Read the model definition and answer for the solid it produces. Units are mm, in the model's axes. Coordinates: 2 decimals unless noted, no trailing zeros. Order: outer loops, then holes, each group sorted by start corner. A loop starts at its lowest first (then second) coordinate and runs counter-clockwise, first axis right, second up. Notation, with made-up numbers: M -3,61.25 L 53,61.25 A22 cw 53,74.25 Z; hole C 7,64 d8. An arc over 180 degrees is marked long. Use a Markdown table: item, result. Add a question column.
1) Find section C-C on x = -18.5. Count the separate pieces of the cut face and the enclosed holes in it, plus the area to 3 significant figures.
2) Find the intervals of material crossed by probe 1 along X at (y, z) = (1.85, -2); probe 2 along X at (y, z) = (0.75, -46.5); probe 3 along Z at (x, y) = (48, 1.7), in increasing order. Write a range as [from, to].
3) Find section A-A on z = 0. Write down the section's boundary in (x, y).
4) Find section B-B on x = -57.5. Write down the section's boundary in (y, z).
5) Each of these flat-tipped pins is pushed along its axis until it touches: pin 1 Ø1 at (x, y) = (22, 1) entering from -Z; pin 2 Ø8 at (x, z) = (-49, 46.5) entering from -Y; pin 3 Ø1 at (y, z) = (1, -41.5) entering from -X; pin 4 Ø1 at (y, z) = (1, 49) entering from -X. Where does it stop, or does it pass through?
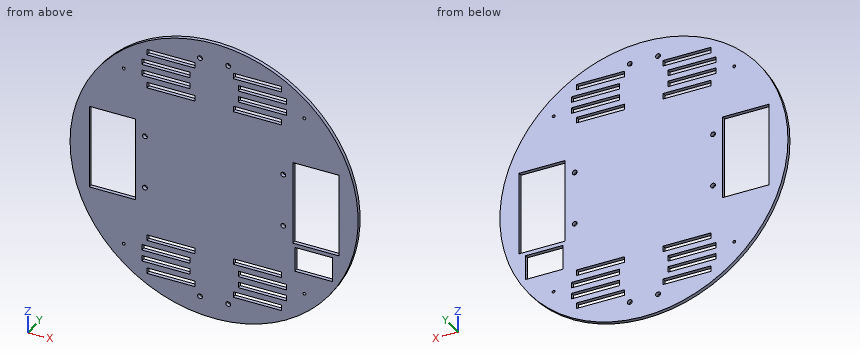
Autodesk Inventor part; units mm, degrees
ref_plane "YZ Plane" through (0, 0, 0) normal (1, 0, 0) x (0, 1, 0)
ref_plane "XZ Plane" through (0, 0, 0) normal (0, 1, 0) x (-1, 0, 0)
ref_plane "XY Plane" through (0, 0, 0) normal (0, 0, 1) x (1, 0, 0)
sketch "Boceto1" plane through (0, 0, 0) normal (0, 1, 0) x (-1, 0, 0)
  circle A0 centre (0, 0) radius 75
  line L0 (65, -22) -> (41, -22)
  line L1 (41, -22) -> (41, 22)
  line L2 (41, 22) -> (65, 22)
  line L3 (65, 22) -> (65, -22)
  line L4 (37.6072, -48.4982) -> (12.6072, -48.4982)
  line L5 (12.6072, -48.4982) -> (12.6072, -45.4982)
  line L6 (12.6072, -45.4982) -> (37.6072, -45.4982)
  line L7 (37.6072, -45.4982) -> (37.6072, -48.4982)
  line L8 (37.6072, -54.4982) -> (12.6072, -54.4982)
  line L9 (12.6072, -54.4982) -> (12.6072, -51.4982)
  line L10 (12.6072, -51.4982) -> (37.6072, -51.4982)
  line L11 (37.6072, -51.4982) -> (37.6072, -54.4982)
  line L12 (35, -60.4982) -> (10, -60.4982)
  line L13 (10, -60.4982) -> (10, -57.4982)
  line L14 (10, -57.4982) -> (35, -57.4982)
  line L15 (35, -57.4982) -> (35, -60.4982)
  line L16 (35, -42.4982) -> (10, -42.4982)
  line L17 (10, -42.4982) -> (10, -39.4982)
  line L18 (10, -39.4982) -> (35, -39.4982)
  line L19 (35, -39.4982) -> (35, -42.4982)
  line L20 (-37.6072, -48.4982) -> (-12.6072, -48.4982)
  line L21 (-12.6072, -48.4982) -> (-12.6072, -45.4982)
  line L22 (-12.6072, -45.4982) -> (-37.6072, -45.4982)
  line L23 (-37.6072, -45.4982) -> (-37.6072, -48.4982)
  line L24 (-37.6072, -54.4982) -> (-12.6072, -54.4982)
  line L25 (-37.6072, -51.4982) -> (-37.6072, -54.4982)
  line L26 (-12.6072, -51.4982) -> (-37.6072, -51.4982)
  line L27 (-12.6072, -54.4982) -> (-12.6072, -51.4982)
  line L28 (-35, -60.4982) -> (-10, -60.4982)
  line L29 (-35, -57.4982) -> (-35, -60.4982)
  line L30 (-10, -57.4982) -> (-35, -57.4982)
  line L31 (-10, -60.4982) -> (-10, -57.4982)
  line L32 (-35, -42.4982) -> (-10, -42.4982)
  line L33 (-35, -39.4982) -> (-35, -42.4982)
  line L34 (-10, -39.4982) -> (-35, -39.4982)
  line L35 (-10, -42.4982) -> (-10, -39.4982)
  line L36 (-65, -22) -> (-41, -22)
  line L37 (-41, -22) -> (-41, 22)
  line L38 (-41, 22) -> (-65, 22)
  line L39 (-65, 22) -> (-65, -22)
  line L40 (37.6072, 49.7986) -> (12.6072, 49.7986)
  line L41 (12.6072, 49.7986) -> (12.6072, 46.7986)
  line L42 (12.6072, 46.7986) -> (37.6072, 46.7986)
  line L43 (37.6072, 46.7986) -> (37.6072, 49.7986)
  line L44 (37.6072, 55.7986) -> (12.6072, 55.7986)
  line L45 (37.6072, 52.7986) -> (37.6072, 55.7986)
  line L46 (12.6072, 52.7986) -> (37.6072, 52.7986)
  line L47 (12.6072, 55.7986) -> (12.6072, 52.7986)
  line L48 (35, 61.7986) -> (10, 61.7986)
  line L49 (35, 58.7986) -> (35, 61.7986)
  line L50 (10, 58.7986) -> (35, 58.7986)
  line L51 (10, 61.7986) -> (10, 58.7986)
  line L52 (35, 43.7986) -> (10, 43.7986)
  line L53 (35, 40.7986) -> (35, 43.7986)
  line L54 (10, 40.7986) -> (35, 40.7986)
  line L55 (10, 43.7986) -> (10, 40.7986)
  line L56 (-35, 40.7986) -> (-35, 43.7986)
  line L57 (-10, 43.7986) -> (-10, 40.7986)
  line L58 (-10, 40.7986) -> (-35, 40.7986)
  line L59 (-35, 43.7986) -> (-10, 43.7986)
  line L60 (-12.6072, 49.7986) -> (-12.6072, 46.7986)
  line L61 (-12.6072, 46.7986) -> (-37.6072, 46.7986)
  line L62 (-37.6072, 46.7986) -> (-37.6072, 49.7986)
  line L63 (-37.6072, 49.7986) -> (-12.6072, 49.7986)
  line L64 (-12.6072, 55.7986) -> (-12.6072, 52.7986)
  line L65 (-12.6072, 52.7986) -> (-37.6072, 52.7986)
  line L66 (-37.6072, 55.7986) -> (-12.6072, 55.7986)
  line L67 (-10, 58.7986) -> (-35, 58.7986)
  line L68 (-35, 61.7986) -> (-10, 61.7986)
  line L69 (-10, 61.7986) -> (-10, 58.7986)
  line L70 (-37.6072, 52.7986) -> (-37.6072, 55.7986)
  line L71 (-35, 58.7986) -> (-35, 61.7986)
  point P0 (0, 25.3749)
  dimension "d0" = 150
  dimension "d1" = 24
  dimension "d2" = 44
  dimension "d3" = 10
  dimension "d4" = 25
  dimension "d5" = 3
  dimension "d6" = 25
  dimension "d7" = 3
  dimension "d8" = 25
  dimension "d9" = 3
  dimension "d10" = 25
  dimension "d11" = 3
  dimension "d12" = 3
  dimension "d13" = 3
  dimension "d14" = 3
  dimension "d15" = 0
extrude "Extrusión1" add sketch "Boceto1" along normal blind 2
sketch "Boceto2" plane through (0, 2, 0) normal (0, 1, 0) x (1, 0, 0)
  line L0 (0, 0) -> (0, -9.9603)
  line L1 (0, 0) -> (61.7788, -62.8893)
  circle A0 centre (47.0174, -47.8626) radius 0.75
  arc A1 (50.5529, -44.327) -> (43.5135, -51.4295) centre (47.0174, -47.8626) ccw
  line L2 (-72.438, 0) -> (-75, 0)
  circle A2 centre (0, 0) radius 72.438
  line L3 (44.0781, -44.8705) -> (47.0174, -47.8626)
  line L4 (43.4505, -51.3665) -> (48.0344, -55.9504)
  line L5 (43.4505, -51.3665) -> (49.9332, -51.3665) construction
  line L6 (47.0174, -47.8626) -> (52.0174, -47.8626) construction
  line L7 (50.5529, -44.327) -> (55.1054, -48.8795)
  line L8 (55.1054, -48.8795) -> (48.0344, -55.9504)
  circle A3 centre (-47.0174, -47.8626) radius 0.75
  arc A4 (-43.5135, -51.4295) -> (-50.5529, -44.327) centre (-47.0174, -47.8626) ccw
  line L9 (-44.0781, -44.8705) -> (-47.0174, -47.8626)
  line L10 (-43.4505, -51.3665) -> (-48.0344, -55.9504)
  line L11 (-43.4505, -51.3665) -> (-49.9332, -51.3665) construction
  line L12 (-47.0174, -47.8626) -> (-52.0174, -47.8626) construction
  line L13 (-50.5529, -44.327) -> (-55.1054, -48.8795)
  line L14 (-55.1054, -48.8795) -> (-48.0344, -55.9504)
  line L15 (0, 0) -> (7.916, 0)
  line L16 (-44.0781, 44.8705) -> (-47.0174, 47.8626)
  circle A5 centre (-47.0174, 47.8626) radius 0.75
  line L17 (-43.4505, 51.3665) -> (-49.9332, 51.3665) construction
  arc A6 (-50.5529, 44.327) -> (-43.5135, 51.4295) centre (-47.0174, 47.8626) ccw
  line L18 (-43.4505, 51.3665) -> (-48.0344, 55.9504)
  line L19 (-47.0174, 47.8626) -> (-52.0174, 47.8626) construction
  line L20 (-50.5529, 44.327) -> (-55.1054, 48.8795)
  line L21 (-55.1054, 48.8795) -> (-48.0344, 55.9504)
  line L22 (0, 0) -> (61.7788, 62.8893)
  circle A7 centre (0, 0) radius 72.438
  circle A8 centre (47.0174, 47.8626) radius 0.75
  arc A9 (43.5135, 51.4295) -> (50.5529, 44.327) centre (47.0174, 47.8626) ccw
  line L23 (44.0781, 44.8705) -> (47.0174, 47.8626)
  line L24 (43.4505, 51.3665) -> (48.0344, 55.9504)
  line L25 (47.0174, 47.8626) -> (52.0174, 47.8626) construction
  line L26 (55.1054, 48.8795) -> (48.0344, 55.9504)
  line L27 (50.5529, 44.327) -> (55.1054, 48.8795)
  line L28 (43.4505, 51.3665) -> (49.9332, 51.3665) construction
  dimension "d26" = 1.5
  dimension "d27" = 45
  dimension "d28" = 44.49
  dimension "d29" = 45.51
extrude "Extrusión2" cut sketch "Boceto2" against normal blind 10 contours A0 L1 | L1 A0 | A8 L22 | L22 A8 | A3 | A5
sketch "Boceto3" plane through (0, 0, 0) normal (0, -1, 0) x (1, 0, 0)
  line L0 (0, 0) -> (0, 96.9999)
  line L1 (0, 0) -> (57.8177, 0)
  circle A0 centre (7.35, 65) radius 1.25
  circle A1 centre (-7.35, 65) radius 1.25
  circle A2 centre (7.35, -65) radius 1.25
  circle A3 centre (-7.35, -65) radius 1.25
  dimension "d32" = 2.5
  dimension "d33" = 7.35
  dimension "d34" = 65
extrude "Extrusión3" cut sketch "Boceto3" against normal blind 10
sketch "Boceto4" plane through (0, 0, 0) normal (0, -1, 0) x (1, 0, 0)
  circle A0 centre (-36, 14) radius 1.25
  line L0 (0, 0) -> (0, 13.2611)
  line L1 (0, 0) -> (12.4525, 0)
  circle A1 centre (36, 14) radius 1.25
  circle A2 centre (-36, -14) radius 1.25
  circle A3 centre (36, -14) radius 1.25
  line L2 (-41, 22) -> (-41, -22)
  point P0 (0, -13.2611)
  dimension "d37" = 2.5
  dimension "d38" = 14
  dimension "d39" = 5
extrude "Extrusión4" cut sketch "Boceto4" against normal blind 10
sketch "Boceto5" plane through (0, 2, 0) normal (0, 1, 0) x (1, 0, 0)
  line L0 (61.5359, 24) -> (61.5359, 37)
  line L1 (61.5359, 37) -> (42.0359, 37)
  line L2 (42.0359, 37) -> (42.0359, 24)
  line L3 (42.0359, 24) -> (61.5359, 24)
  line L4 (37.6072, 48.4982) -> (37.6072, 45.4982)
  line L5 (41, 22) -> (65, 22)
  point P0 (0, 0)
  dimension "d46" = 13
  dimension "d47" = 19.5
  dimension "d50" = 2
extrude "Extrusión5" cut sketch "Boceto5" against normal blind 10
sketch "Boceto6" plane through (0, 2, 0) normal (0, 1, 0) x (1, 0, 0)
  circle A0 centre (23, 0) radius 0.75
  circle A1 centre (-23, 0) radius 0.75
  line L0 (-20, 33) -> (20, 33)
  line L1 (20, 33) -> (20, -33)
  line L2 (20, -33) -> (-20, -33)
  line L3 (-20, -33) -> (-20, 33)
  circle A2 centre (-23, 32) radius 0.75
  circle A3 centre (-23, -32) radius 0.75
  circle A4 centre (23, -32) radius 0.75
  circle A5 centre (23, 32) radius 0.75
  line L4 (22, 2.2913) -> (22, 29.7087)
  arc A6 (22, 29.7087) -> (22, 34.2913) centre (23, 32) ccw
  line L5 (22, 34.2913) -> (22, 35)
  line L6 (22, 35) -> (-22, 35)
  line L7 (-22, 35) -> (-22, 34.2913)
  arc A7 (-22, 34.2913) -> (-22, 29.7087) centre (-23, 32) ccw
  line L8 (-22, 29.7087) -> (-22, 2.2913)
  arc A8 (-22, 2.2913) -> (-22, -2.2913) centre (-23, 0) ccw
  line L9 (-22, -2.2913) -> (-22, -29.7087)
  arc A9 (-22, -29.7087) -> (-22, -34.2913) centre (-23, -32) ccw
  line L10 (-22, -34.2913) -> (-22, -35)
  line L11 (-22, -35) -> (22, -35)
  line L12 (22, -35) -> (22, -34.2913)
  arc A10 (22, -34.2913) -> (22, -29.7087) centre (23, -32) ccw
  line L13 (22, -29.7087) -> (22, -2.2913)
  arc A11 (22, -2.2913) -> (22, 2.2913) centre (23, 0) ccw
  line L14 (22, -29.7087) -> (22, -34.2913)
  line L15 (-22, -34.2913) -> (-22, -29.7087)
  line L16 (-22, 29.7087) -> (-22, 34.2913)
  line L17 (22, 34.2913) -> (22, 29.7087)
  line L18 (22, -35) -> (-22, -35)
  line L19 (-22, -35) -> (-22, -37)
  line L20 (-22, -37) -> (22, -37)
  line L21 (22, -37) -> (22, -35)
  line L22 (-22, 35) -> (22, 35)
  line L23 (22, 35) -> (22, 37)
  line L24 (22, 37) -> (-22, 37)
  line L25 (-22, 37) -> (-22, 35)
  point P0 (0, 0)
  point P1 (0, 0)
  dimension "d55" = 70
  dimension "d56" = 2
  dimension "d57" = 44
  dimension "d58" = 2
extrude "Extrusión6" [suppressed]
feature "Engrosado1" [suppressed]
properties part number "Base"
Check result:
| question | item | result |
|---|---|---|
| 1 | separate pieces | 9 |
| 1 | enclosed holes | 0 |
| 1 | area | 243 mm2 |
| 2 | probe 1 | x = [-74.97, -65], [-41, 41], [65, 74.97] |
| 2 | probe 2 | x = [-58.85, -37.61], [-12.61, 12.61], [37.61, 58.85] |
| 2 | probe 3 | z = [-57.63, -37], [-24, -22], [22, 57.63] |
| 3 | outline | M -75,0 L -65,0 L -65,2 L -75,2 Z; M -41,0 L 41,0 L 41,2 L -41,2 Z; M 65,0 L 75,0 L 75,2 L 65,2 Z |
| 4 | outline | M 0,-48.15 L 2,-48.15 L 2,-22 L 0,-22 Z; M 0,22 L 2,22 L 2,48.15 L 0,48.15 Z |
| 5 | pin 1 | stops at z = -71.85 |
| 5 | pin 2 | stops at y = 0 |
| 5 | pin 3 | stops at x = -62.8 |
| 5 | pin 4 | stops at x = -57.21 |
